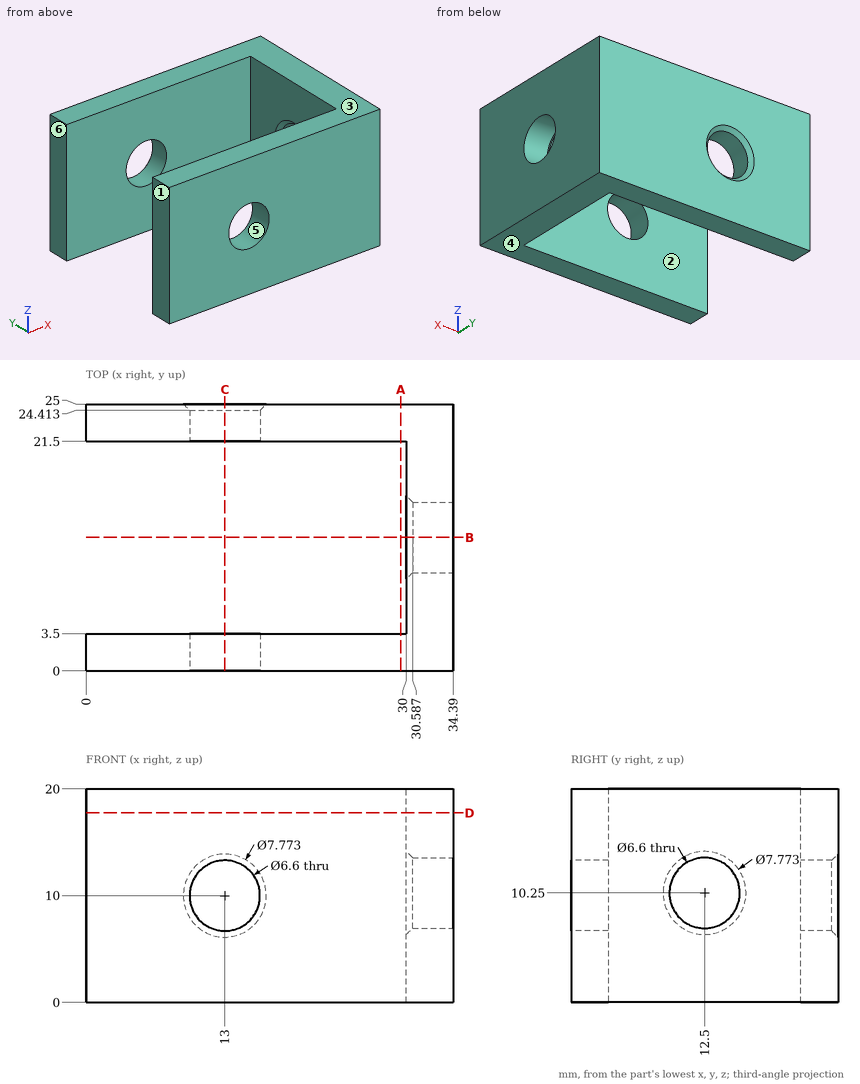
Could you check a few things on this drawing? It's one solid part, dimensions in mm from its lowest x, y, z. A direction names the side the tool comes from. Coordinates: 2 decimals unless noted, no trailing zeros. Write each loop counter-clockwise with the first axis right and the second up, starting at its lowest first coordinate (ties: lowest second). Pieces come first, ordered by that corner, then holes. Notation, with made-up numbers: M -11,4.25 L 35,4.25 A27 ccw 35,43.25 Z; hole C -13,-25 d10. An arc over 180 degrees is marked long. One line per question, with ' | ' between items.
1) Imagine slicing it at D-D, the plane z = 17.75. Write out the boundary of the cut face in (x, y), and give its area (3 significant figures).
Checks:
outline: M 0,0 L 34.39,0 L 34.39,25 L 0,25 L 0,21.5 L 30,21.5 L 30,3.5 L 0,3.5 Z | area: 320 mm²
2) Imagine slicing it at B-B, the plane y = 12.5. Write out the boundary of the cut face in (x, z).
Checks:
outline: M 30,0 L 34.39,0 L 34.39,6.95 L 30.59,6.95 L 30,6.36 Z; M 30,14.14 L 30.59,13.55 L 34.39,13.55 L 34.39,20 L 30,20 Z
3) Imagine slicing it at C-C, the plane x = 13. Write out the boundary of the cut face in (y, z).
Checks:
outline: M 0,0 L 3.5,0 L 3.5,6.7 L 0,6.7 Z; M 0,13.3 L 3.5,13.3 L 3.5,20 L 0,20 Z; M 21.5,0 L 25,0 L 25,6.11 L 24.41,6.7 L 21.5,6.7 Z; M 21.5,13.3 L 24.41,13.3 L 25,13.89 L 25,20 L 21.5,20 Z
4) For the marked faces 1 and 2, which set-ups out of +Z, -Z, +X, -X, +Y, -Y let a thin tool reach every point of the face, with its end or its side?
Checks:
face 1: +Z, -Z, -X, +Y, -Y | face 2: +Z, -Z, -X
5) For pin 1 Ø1 at (x, z) = (20.5, 4) entering from -Y; pin 2 Ø9 at (y, z) = (8.5, 9) entering from -X, each with a flat end and sliding along its axis, tell me the tip position at first contact or that it passes through.
Checks:
pin 1: y = 0 | pin 2: x = 30
6) If we mould it in two halves opening along Z, with no side actions, what happens to the marked faces 3, 4, 5 and 6? For each: released by +Z, released by -Z, zero draft, split by the parting line, or undercut.
Checks:
face 3: released by +Z | face 4: released by -Z | face 5: undercut | face 6: zero draft
7) I need wall thicknesses on probe 1 along Y at (x, z) = (18.5, 2.25); probe 2 along Z at (x, y) = (13, 22.9); probe 3 along X at (y, z) = (22.7, 10). Which ranges of each line are inside material? Lowest first, please. Write a range as [from, to].
Checks:
probe 1: [0, 3.5], [21.5, 25] | probe 2: [0, 6.7], [13.3, 20] | probe 3: [0, 9.7], [16.3, 34.39]
8) Imagine slicing it at A-A, the plane x = 29.5. Write out the boundary of the cut face in (y, z), and give its area (3 significant figures).
Checks:
outline: M 0,0 L 3.5,0 L 3.5,20 L 0,20 Z; M 21.5,0 L 25,0 L 25,20 L 21.5,20 Z | area: 140 mm²
